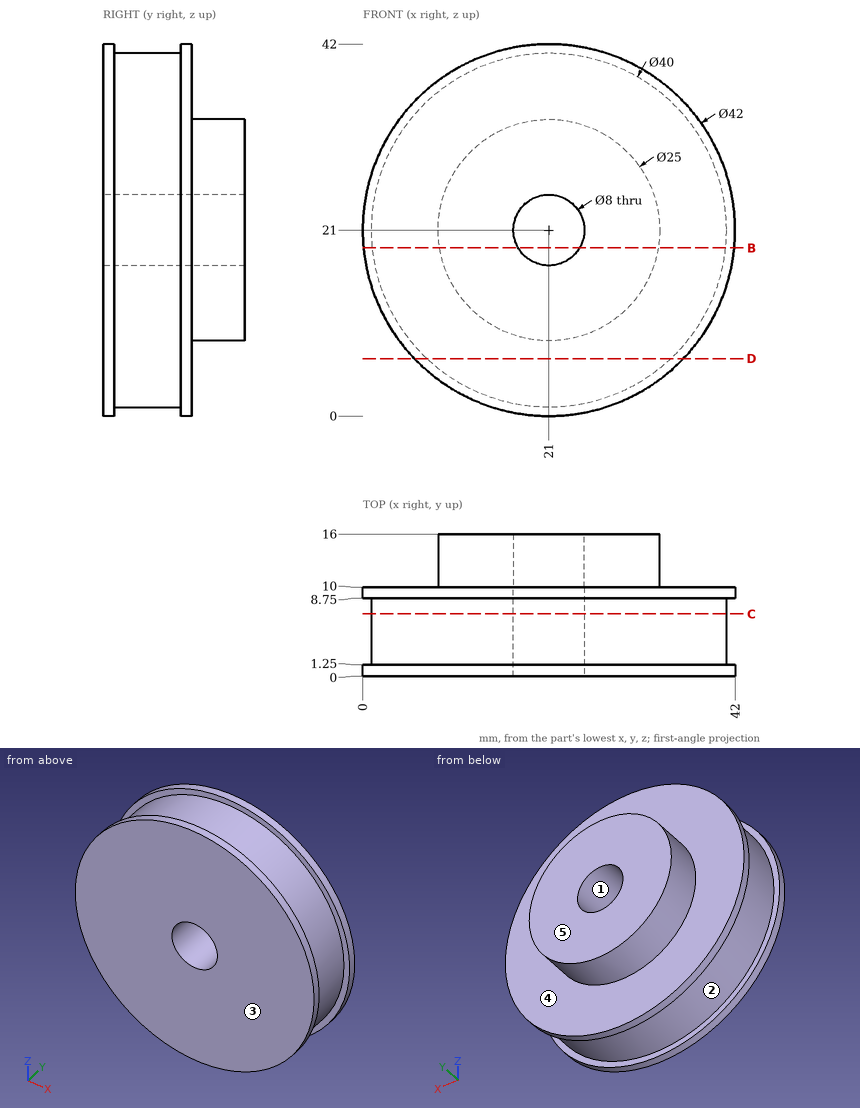
The drawing under review shows one solid part. Ordinate dimensions are in mm from its lowest x, y, z. A direction names the side the tool comes from. Round coordinates to 2 decimals unless told otherwise and drop trailing zeros. Write each loop counter-clockwise with the first axis right and the second up, starting at its lowest first coordinate (ties: lowest second). Pieces come first, ordered by that corner, then holes. Notation, with made-up numbers: (72, -24) -> (103, -24) arc R15 cw to (103, 2) -> close; hole circle Ø10 at (-1, 53.5). An arc over 180 degrees is marked (long way). One line per question, with ' | ' between items. Start each with the question number.
(1) Mouldability with a two-part tool opening along Z and no side actions: class the marked faces 1, 2 and 3 as released by +Z, released by -Z, zero draft, split by the parting line, or undercut.
(2) Add section D-D, the plane z = 6.5. Write out the cut boundary in (x, y), plus the area to 3 significant figures.
(3) Tool access review of the marked faces 4 and 5: name each direction out of +Z, -Z, +X, -X, +Y, -Y from which nothing blocks a thin tool from reaching the whole face with its end or side.
(4) Insertion check: P1, Ø8, axis at y = 7.5, z = 12, coming from the +X side; P2, Ø5, axis at x = 18, z = 15.5, coming from the -Y side; P3, Ø2, axis at y = 13, z = 16.5, coming from the -X side; P4, Ø3, axis at x = 7, y = 7.5, coming from the -Z side. Each pin has a flat end and moves straight along its axis. Give the tip position at first contact, or say it passes through.
(5) For line 1 along X through (y, z) = (4, 21); line 2 along Y through (x, z) = (36.5, 25.5), list the stretches that pass through material, from the lowest coordinate up. Write a range as from..to.
(6) Add section B-B, the plane z = 19. Write out the cut boundary in (x, y).
(7) Add section C-C, the plane y = 7. Write out the cut boundary in (x, z), plus the area to 3 significant figures.
Answer list:
1) face 1: undercut | face 2: split by the parting line | face 3: zero draft
2) outline: (5.81, 0) -> (36.19, 0) -> (36.19, 1.25) -> (34.77, 1.25) -> (34.77, 8.75) -> (36.19, 8.75) -> (36.19, 10) -> (5.81, 10) -> (5.81, 8.75) -> (7.23, 8.75) -> (7.23, 1.25) -> (5.81, 1.25) -> close | area: 283 mm²
3) face 4: +Y | face 5: +Z, -Z, +X, -X, +Y
4) P1: x = 41.35 | P2: y = 0 | P3: x = 9 | P4: z = 4.64
5) line 1: 1..17, 25..41 | line 2: 0..10
6) outline: (0.1, 0) -> (17.54, 0) -> (17.54, 16) -> (8.66, 16) -> (8.66, 10) -> (0.1, 10) -> (0.1, 8.75) -> (1.1, 8.75) -> (1.1, 1.25) -> (0.1, 1.25) -> close; (24.46, 0) -> (41.9, 0) -> (41.9, 1.25) -> (40.9, 1.25) -> (40.9, 8.75) -> (41.9, 8.75) -> (41.9, 10) -> (33.34, 10) -> (33.34, 16) -> (24.46, 16) -> close
7) outline: circle Ø40 at (21, 21); hole circle Ø8 at (21, 21) | area: 1,210 mm²
